The listing builds one solid part. Answer for the finished solid, in the listing's coordinates (mm). A direction names the side the tool comes from. Give positions to 0.01 mm unless a question says otherwise; leave off trailing zeros. Loops run counter-clockwise (first coordinate to the right, second up) from the corner with the lowest first, then second, coordinate; pieces in that order, holes last. Notation, with made-up numbers: M -7.75,19 L 23.25,19 A28 ccw 23.25,48 Z; hole C -15,24 d8. An arc over 180 degrees is marked long. One line per item, written item: value. Start each with the question number.
Q1. For faces 4 (the flat face through (-36, 2, 12.5)), 5 (the flat face through (-35, 22, -1)), 6 (the flat face through (-37.8, 2, -32)), determine the directions among +Z, -Z, +X, -X, +Y, -Y from which every point of the face is accessible in a straight line to the end or side of a thin tool.
Q2. A cutting plane is placed at A-A, the plane z = 0. Determine the outline of the cut face in (x, y), and give its area (3 significant figures).
Q3. Consider L1, parallel to Z at x = -31, y = 3; L2, parallel to X at y = 10.5, z = 37.5; L3, parallel to Z at x = -4.5, y = 25. Determine where each line is inside the solid, lowest interval first.
Q4. Flat-ended cylindrical pins translate along their axes: pin 1 (1.2 mm diameter, centred on x = 13, y = 2, fed in from -Z); pin 2 (4.5 mm diameter, centred on y = 1, z = 37, fed in from -X); pin 3 (2 mm diameter, centred on x = 7, y = 1.5, fed in from +Z). Find the tip coordinate at first contact, or state that the pin passes through.
Q5. The mould has two halves that part along X. Classify faces 1 (the flat face through (35, 22, -1)), 2 (the flat face through (-37.8, 2, 31)), 3 (the flat face through (0, 4, -52)): +X half, -X half, draft (parallel to the pull), parting line (faces both ways), or undercut.
Q6. A cutting plane is placed at C-C, the plane x = -14.5. Determine the outline of the cut face in (y, z).
Q7. A cutting plane is placed at D-D, the plane y = 40.5. Determine the outline of the cut face in (x, z).
Q8. A cutting plane is placed at B-B, the plane y = 12.5. Determine the outline of the cut face in (x, z), and give its area (3 significant figures).
from build123d import *

# Parameters (mm, degrees)
SKETCH1_W           = 80
SKETCH1_H           = 105
BOSS_EXTRUDE1_DEPTH = 48
SKETCH3_W           = 70
SKETCH3_H           = 95
CUT_EXTRUDE1_DEPTH  = 45
SKETCH4_W           = 80
SKETCH4_H           = 105
SKETCH4_W_2         = 75.6
SKETCH4_H_2         = 100.6
CUT_EXTRUDE2_DEPTH  = 4
CUT_EXTRUDE3_DEPTH  = 108.052557186


with BuildPart() as part:
    # Sketch1 → Boss-Extrude1 (new body)
    with BuildSketch(Plane(origin=(0, 0, 0), x_dir=(1, 0, 0), z_dir=(0, 1, 0))):
        Rectangle(SKETCH1_W, SKETCH1_H)
    extrude(amount=BOSS_EXTRUDE1_DEPTH)

    # Sketch3 → Cut-Extrude1 (cut)
    with BuildSketch(Plane.XZ):
        Rectangle(SKETCH3_W, SKETCH3_H)
    extrude(amount=-CUT_EXTRUDE1_DEPTH, mode=Mode.SUBTRACT)

    # Sketch4 → Cut-Extrude2 (cut)
    with BuildSketch(Plane.XZ):
        Rectangle(SKETCH4_W, SKETCH4_H)
        Rectangle(SKETCH4_W_2, SKETCH4_H_2, mode=Mode.SUBTRACT)
    extrude(amount=-CUT_EXTRUDE2_DEPTH, mode=Mode.SUBTRACT)

    # Sketch5 → Cut-Extrude3 (cut, through all)
    with BuildSketch(Plane(origin=(40, 0, 0), x_dir=(0, 0, -1), z_dir=(1, 0, 0))):
        with BuildLine():
            Line((-12.5, 4), (-12.5, -5.5))
            Line((-12.5, -5.5), (12.5, -5.5))
            Line((12.5, -5.5), (12.5, 4))
            ThreePointArc((12.5, 4), (0, 16.5), (-12.5, 4))
        make_face()
    extrude(amount=-CUT_EXTRUDE3_DEPTH, mode=Mode.SUBTRACT)


solid = part.part
Answer block:
1. face 4: +X, -X, -Y
1. face 5: -Y
1. face 6: +Z, -Z, -X, -Y
2. outline: M -40,16.5 L -35,16.5 L -35,45 L 35,45 L 35,16.5 L 40,16.5 L 40,48 L -40,48 Z
2. area: 525 mm^2
3. L1: -50.3 to -47.5, 47.5 to 50.3
3. L2: -40 to -35, 35 to 40
3. L3: -52.5 to -47.5, 47.5 to 52.5
4. pin 1: z = -50.3
4. pin 2: x = -37.8
4. pin 3: z = 50.3
5. face 1: undercut
5. face 2: -X half
5. face 3: draft
6. outline: M 0,-50.3 L 4,-50.3 L 4,-52.5 L 48,-52.5 L 48,52.5 L 4,52.5 L 4,50.3 L 0,50.3 L 0,47.5 L 45,47.5 L 45,-47.5 L 0,-47.5 Z
7. outline: M -40,-52.5 L 40,-52.5 L 40,52.5 L -40,52.5 Z; hole M -35,-47.5 L 35,-47.5 L 35,47.5 L -35,47.5 Z
8. outline: M -40,-52.5 L 40,-52.5 L 40,-9.17 L 35,-9.17 L 35,-47.5 L -35,-47.5 L -35,-9.17 L -40,-9.17 Z; M -40,9.17 L -35,9.17 L -35,47.5 L 35,47.5 L 35,9.17 L 40,9.17 L 40,52.5 L -40,52.5 Z
8. area: 1,570 mm^2
